Verification items for the finished model (mm, model axes). Face numbers are marked on the shaded views. A direction names the side the tool comes from. Coordinates: 2 decimals unless noted, no trailing zeros. Order: outer loops, then holes, each group sorted by start corner. A loop starts at its lowest first (then second) coordinate and runs counter-clockwise, first axis right, second up. Notation, with made-up numbers: (16, -14) -> (74, -14) arc R22 ccw to (74, 12) -> close; hole circle Ø6 at (48.25, 69.5). An arc over 180 degrees is marked (long way). Answer as CSV lines item,"result".
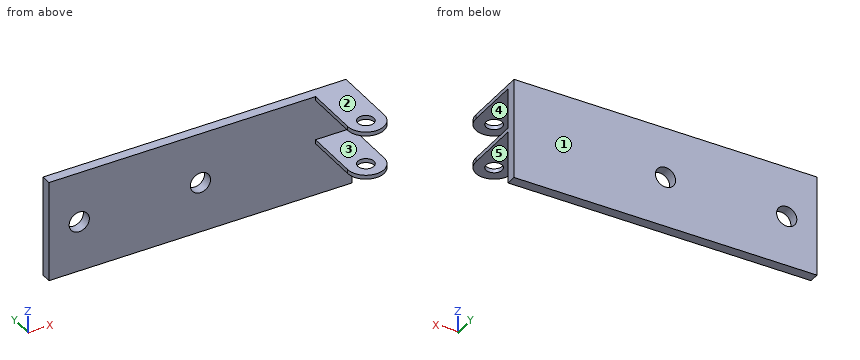
Autodesk Inventor part; units mm, degrees
ref_plane "YZ Plane" through (0, 0, 0) normal (1, 0, 0) x (0, 1, 0)
ref_plane "XZ Plane" through (0, 0, 0) normal (0, 1, 0) x (-1, 0, 0)
ref_plane "XY Plane" through (0, 0, 0) normal (0, 0, 1) x (1, 0, 0)
sketch "Sketch1" plane through (0, 0, 0) normal (0, 1, 0) x (-1, 0, 0)
  line L0 (0, 0) -> (150, 0)
  line L1 (150, 0) -> (150, -50)
  line L2 (150, -50) -> (0, -50)
  line L3 (0, -50) -> (0, 0)
  dimension "d0" = 150
  dimension "d1" = 50
extrude "Extrusion1" add sketch "Sketch1" along normal blind 5
sketch "Sketch2" plane through (0, 5, 0) normal (0, 1, 0) x (1, 0, 0)
  circle A0 centre (-135, 25) radius 5
  line L0 (-150, 0) -> (0, 0)
  line L1 (-150, 50) -> (-150, 0)
  circle A1 centre (-75, 25) radius 5
  dimension "d4" = 10
  dimension "d5" = 25
  dimension "d6" = 15
  dimension "d7" = 10
  dimension "d8" = 25
  dimension "d9" = 60
extrude "Extrusion2" cut sketch "Sketch2" against normal blind 5
sketch "Sketch4" plane through (0, 0, 0) normal (0, -1, 0) x (1, 0, 0)
  line L0 (0, 0) -> (0, -50)
  line L1 (0, 0) -> (-18, 0)
  line L2 (-18, 0) -> (-18, -2)
  line L3 (-18, -2) -> (0, -2)
  line L4 (0, -2) -> (0, 0)
  line L5 (0, -22) -> (-18, -22)
  line L6 (-18, -22) -> (-18, -24)
  line L7 (-18, -24) -> (0, -24)
  line L8 (0, -24) -> (0, -22)
  dimension "d17" = 18
  dimension "d18" = 2
  dimension "d19" = 18
  dimension "d20" = 2
  dimension "d21" = 20
extrude "Extrusion4" add sketch "Sketch4" along normal blind 36
sketch "Sketch5" plane through (-150, 5, 0) normal (0, 0, 1) x (1, 0, 0)
  circle A0 centre (141, -32) radius 9
  line L0 (150, -41) -> (150, 0)
  line L1 (150, -41) -> (132, -41)
  line L2 (150, -32) -> (150, -41)
  line L3 (132, -41) -> (132, -32)
  line L4 (132, -5) -> (132, -41)
  line L5 (132, -41) -> (150, -41)
  circle A1 centre (141, -32) radius 4
  point P0 (150, -5)
  dimension "d24" = 18
  dimension "d25" = 9
  dimension "d26" = 9
  dimension "d27" = 8
extrude "Extrusion5" cut sketch "Sketch5" against normal blind 36 contours L0 L1 A0 | A0 L1 L3 | A1
properties part number "Giá đỡ ròng rọc 2"
Item 1: Section check B-B, the plane x = -135. Record the boundary of the cut face in (y, z).
Answer list:
outline,"(0, -50) -> (5, -50) -> (5, -30) -> (0, -30) -> close; (0, -20) -> (5, -20) -> (5, 0) -> (0, 0) -> close"
Item 2: Section check A-A, the plane x = -9. Record the boundary of the cut face in (y, z).
Answer list:
outline,"(-36, -24) -> (-31, -24) -> (-31, -22) -> (-36, -22) -> close; (-36, -2) -> (-31, -2) -> (-31, 0) -> (-36, 0) -> close; (-23, -24) -> (0, -24) -> (0, -50) -> (5, -50) -> (5, 0) -> (-23, 0) -> (-23, -2) -> (0, -2) -> (0, -22) -> (-23, -22) -> close"
Item 3: Depth check by flat-ended pin: pin 1 Ø5.5 at (x, y) = (-11.5, -25) entering from -Z; pin 2 Ø1 at (y, z) = (-16.5, -1) entering from -X; pin 3 Ø5 at (x, y) = (-9, -27) entering from +Z; pin 4 Ø20 at (x, y) = (-11.5, -20.5) entering from +Z. Enter the tip coordinate at first touch or a pass-through.
Answer list:
pin 1,"z = -24"
pin 2,"x = -18"
pin 3,"through"
pin 4,"z = 0"
Item 4: Thickness scan on line 1 (X direction, y = 2.35, z = -25); line 2 (Z direction, x = -75, y = 3); line 3 (Z direction, x = -6, y = -12). Record the ranges inside material, lowest first.
Answer list:
line 1,"-150 to -140, -130 to -80, -70 to 0"
line 2,"-50 to -30, -20 to 0"
line 3,"-24 to -22, -2 to 0"
Item 5: Release check for a two-part mould opening along Z. For the marked faces 1, 2 and 3 record: +Z half, -Z half, draft (parallel to the pull), parting line (faces both ways), or undercut.
Answer list:
face 1,"draft"
face 2,"+Z half"
face 3,"undercut"
Item 6: Tool access check on the marked faces 4 and 5. Record the directions out of +Z, -Z, +X, -X, +Y, -Y that give a thin tool (end or side, any length) a straight path to the whole face; none if there is none.
Answer list:
face 4,"+X, -X, -Y"
face 5,"-Z, +X, -X, -Y"
Item 7: Section check D-D, the plane y = 2. Record the boundary of the cut face in (x, z), plus the area to 3 significant figures.
Answer list:
outline,"(-150, -50) -> (0, -50) -> (0, 0) -> (-150, 0) -> close; hole circle Ø10 at (-135, -25); hole circle Ø10 at (-75, -25)"
area,"7,340 mm2"
Item 8: Section check C-C, the plane y = -19. Record the boundary of the cut face in (x, z), plus the area to 3 significant figures.
Answer list:
outline,"(-18, -24) -> (0, -24) -> (0, -22) -> (-18, -22) -> close; (-18, -2) -> (0, -2) -> (0, 0) -> (-18, 0) -> close"
area,"72.0 mm2"
